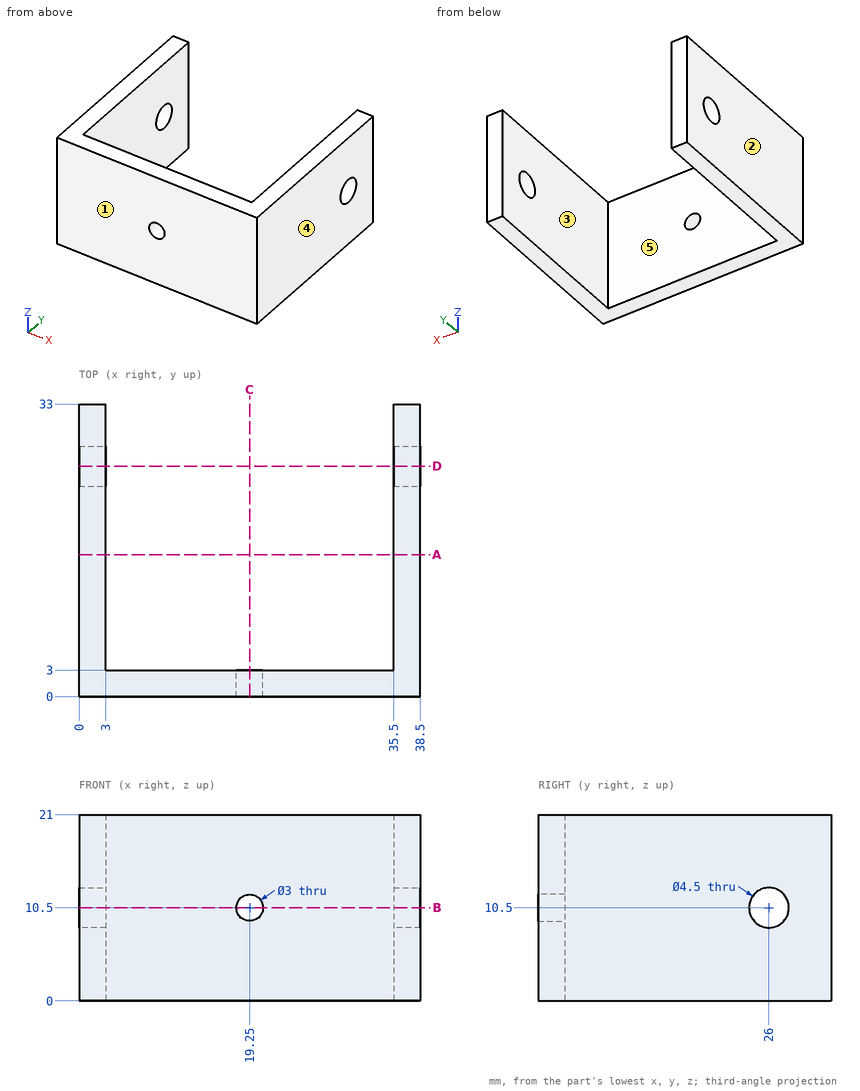
For this review, use the dimensioned drawing (mm, ordinates from the lowest corner) and the shaded views. A direction names the side the tool comes from. Give positions to 0.01 mm unless a question says otherwise; leave off trailing zeros. Order: outer loops, then holes, each group sorted by start corner. A loop starts at its lowest first (then second) coordinate and runs counter-clockwise, first axis right, second up.
1. To check wall thickness, follow L1, parallel to X at y = 0.9, z = 10.5; L2, parallel to X at y = 11, z = 20.25; L3, parallel to Y at x = 1.2, z = 10.5. State the ranges of each line that lie inside material, in increasing order.
Solution:
L1: x = 0 to 17.75, 20.75 to 38.5
L2: x = 0 to 3, 35.5 to 38.5
L3: y = 0 to 23.75, 28.25 to 33
2. Add section C-C, the plane x = 19.25. State the section outline as (y, z) points.
Solution:
outline: (0, 0) - (3, 0) - (3, 9) - (0, 9) - close; (0, 12) - (3, 12) - (3, 21) - (0, 21) - close
3. Add section B-B, the plane z = 10.5. State the section outline as (x, y) points, then the cut area to 4 significant figures.
Solution:
outline: (0, 0) - (17.75, 0) - (17.75, 3) - (3, 3) - (3, 23.75) - (0, 23.75) - close; (0, 28.25) - (3, 28.25) - (3, 33) - (0, 33) - close; (20.75, 0) - (38.5, 0) - (38.5, 23.75) - (35.5, 23.75) - (35.5, 3) - (20.75, 3) - close; (35.5, 28.25) - (38.5, 28.25) - (38.5, 33) - (35.5, 33) - close
area: 259.5 mm2
4. Tool access review of the marked faces 4 and 5: name each direction out of +Z, -Z, +X, -X, +Y, -Y from which nothing blocks a thin tool from reaching the whole face with its end or side.
Solution:
face 4: +Z, -Z, +X, +Y, -Y
face 5: +Z, -Z, +Y
5. Add section A-A, the plane y = 16. State the section outline as (x, z) points.
Solution:
outline: (0, 0) - (3, 0) - (3, 21) - (0, 21) - close; (35.5, 0) - (38.5, 0) - (38.5, 21) - (35.5, 21) - close
6. For pin 1 Ø7 at (y, z) = (26, 10.5) entering from -X; pin 2 Ø1 at (x, z) = (13, 10) entering from +Y; pin 3 Ø2.5 at (x, z) = (19.25, 10.5) entering from -Y, all flat-tipped, find the tip position at first contact; note any pin that passes through.
Solution:
pin 1: stops at x = 0
pin 2: stops at y = 3
pin 3: passes through
7. Mouldability with a two-part tool opening along X and no side actions: class the marked faces 1, 2 and 3 as +X half, -X half, draft (parallel to the pull), parting line (faces both ways), or undercut.
Solution:
face 1: draft
face 2: -X half
face 3: undercut
8. Add section D-D, the plane y = 26. State the section outline as (x, z) points.
Solution:
outline: (0, 0) - (3, 0) - (3, 8.25) - (0, 8.25) - close; (0, 12.75) - (3, 12.75) - (3, 21) - (0, 21) - close; (35.5, 0) - (38.5, 0) - (38.5, 8.25) - (35.5, 8.25) - close; (35.5, 12.75) - (38.5, 12.75) - (38.5, 21) - (35.5, 21) - close
